```python
from build123d import *

# Parameters (mm, degrees)
F0_R     = 15
F0_W     = 10
F0_H     = 15
F1_DEPTH = 75
F2_R     = 5
F3_DEPTH = 50.001
F4_R     = 10
F5_DEPTH = 10.001


with BuildPart() as f1:
    # F0 (on Front) → F1 (new body)
    with BuildSketch(Plane.XZ):
        with BuildLine():
            Line((60, -2.5), (60, 12.5))
            Line((60, 12.5), (-15, 12.5))
            ThreePointArc((-15, 12.5), (-29.142136, 6.642136), (-35, -7.5))
            Line((-35, -7.5), (-35, -22.5))
            Line((-35, -22.5), (-50, -22.5))
            Line((-50, -22.5), (-50, -37.5))
            Line((-50, -37.5), (-5, -37.5))
            ThreePointArc((-5, -37.5), (9.142136, -31.642136), (15, -17.5))
            Line((15, -17.5), (15, -2.5))
            Line((15, -2.5), (60, -2.5))
        make_face()
        with Locations((-10, -12.5)):
            Circle(F0_R, mode=Mode.SUBTRACT)
        Polygon((-50, -22.5), (-50, 22.5), (-60, 22.5), (-60, -37.5), (-50, -37.5), align=None)
        with Locations((-55, 30)):
            Rectangle(F0_W, F0_H)
    extrude(amount=F1_DEPTH)

    # F2 (on face) → F3 (cut, through all)
    with BuildSketch(Plane.XY.offset(12.5)):
        with Locations((45, -20)):
            Circle(F2_R)
        with Locations((45, -55)):
            Circle(F2_R)
    extrude(amount=-F3_DEPTH, mode=Mode.SUBTRACT)

    # F4 (on face) → F5 (cut, through all)
    with BuildSketch(Plane.YZ.offset(-50)):
        with Locations((-40, 2.5)):
            Circle(F4_R)
        Polygon((-75, 37.5), (-75, 22.5), (-60, 37.5), align=None)
        Polygon((0, 37.5), (-15, 37.5), (0, 22.5), align=None)
    extrude(amount=-F5_DEPTH, mode=Mode.SUBTRACT)


solid = f1.part
```
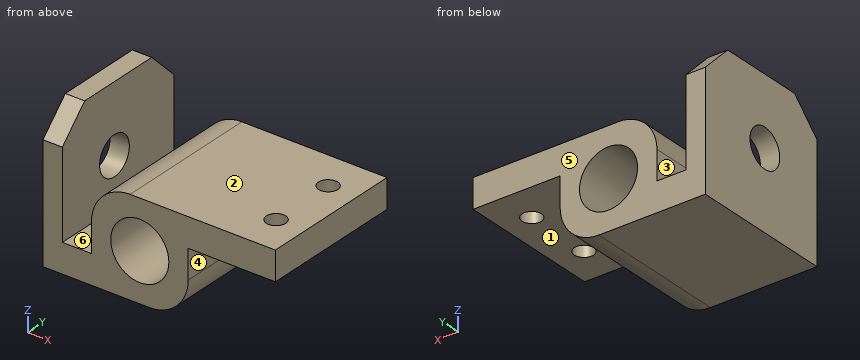
Check sheet for the modelled part. Datum: model origin and axes. Units: mm. Face numbers are marked on the shaded views. A direction names the side the tool comes from. Give positions to 0.01 mm unless a question says otherwise; leave off trailing zeros. Order: outer loops, then holes, each group sorted by start corner. A loop starts at its lowest first (then second) coordinate and runs counter-clockwise, first axis right, second up. Notation, with made-up numbers: M 14,8 L 63,8 A23 cw 63,27 Z; hole C 21,16 d1. An arc over 180 degrees is marked long. Answer in a Markdown table with one row per item. Add a question column.
Q1. Release check for a two-part mould opening along X. For the marked faces 4, 5 and 6 record: released by +X, released by -X, zero draft, split by the parting line, or undercut.
Q2. Access from +Z, -Z, +X, -X, +Y, -Y to the whole of each face (thin tool, end or side, straight path). Record for the marked faces 1, 2 and 3.
Q3. Sectioned sample at D-D, the plane z = -12.5. Record the boundary of the cut face in (x, y), and give its area (3 significant figures).
Q4. Sectioned sample at B-B, the plane x = -10. Record the boundary of the cut face in (y, z).
Q5. Thickness scan on L1, parallel to X at y = -22.5, z = -8.5; L2, parallel to Z at x = -10, y = -41; L3, parallel to X at y = -47, z = -10.5. Record the ranges inside material, lowest first.
Q6. Gauge pin test, flat ends, axial feed: pin 1 Ø11.5 at (x, y) = (45, -20) entering from +Z; pin 2 Ø4.5 at (y, z) = (-39, -8) entering from +X; pin 3 Ø7.5 at (x, y) = (-43.5, -36) entering from +Z. Record the tip position at first contact, or that the pin passes through.
Q7. Sectioned sample at C-C, the plane z = 9. Record the boundary of the cut face in (x, y).
Q8. Sectioned sample at A-A, the plane y = -55. Record the boundary of the cut face in (x, z), and give its area (3 significant figures).
Verdict:
| question | item | result |
|---|---|---|
| 1 | face 4 | released by +X |
| 1 | face 5 | zero draft |
| 1 | face 6 | undercut |
| 2 | face 1 | -Z, +X, +Y, -Y |
| 2 | face 2 | +Z, +X, +Y, -Y |
| 2 | face 3 | +Z, +Y, -Y |
| 3 | outline | M -60,-75 L -50,-75 L -50,0 L -60,0 Z; M -35,-75 L -25,-75 L -25,0 L -35,0 Z; M 5,-75 L 15,-75 L 15,0 L 5,0 Z |
| 3 | area | 2,250 mm² |
| 4 | outline | M -75,-37.5 L 0,-37.5 L 0,-27.5 L -75,-27.5 Z; M -75,2.5 L 0,2.5 L 0,12.5 L -75,12.5 Z |
| 5 | L1 | -60 to -50, -35 to -24.46, 4.46 to 15 |
| 5 | L2 | -37.5 to -27.5, 2.5 to 12.5 |
| 5 | L3 | -60 to -50, -35 to -24.87, 4.87 to 15 |
| 6 | pin 1 | z = 12.5 |
| 6 | pin 2 | x = 15 |
| 6 | pin 3 | z = -22.5 |
| 7 | outline | M -60,-75 L -50,-75 L -50,-47.6 L -60,-47.6 Z; M -60,-32.4 L -50,-32.4 L -50,0 L -60,0 Z; M -26.3,-75 L 60,-75 L 60,0 L -26.3,0 Z; hole C 45,-55 d10; hole C 45,-20 d10 |
| 8 | outline | M -60,-37.5 L -5,-37.5 A20 ccw 15,-17.5 L 15,-2.5 L 40,-2.5 L 40,12.5 L -15,12.5 A20 ccw -35,-7.5 L -35,-22.5 L -50,-22.5 L -50,37.5 L -60,37.5 Z; M 50,-2.5 L 60,-2.5 L 60,12.5 L 50,12.5 Z; hole C -10,-12.5 d30 |
| 8 | area | 3,120 mm² |
